Input: dimensioned drawing with shaded views. Units: mm. Origin: part minimum x, y, z. A direction names the side the tool comes from. Give positions to 0.01 mm unless a question says otherwise; leave off trailing zeros. Order: outer loops, then holes, each group sorted by start corner. A loop starts at its lowest first (then second) coordinate and runs counter-clockwise, first axis right, second up. Notation, with made-up numbers: (-25, 89.25) -> (9, 89.25) arc R24 cw to (9, 128.25) -> close; hole circle Ø6 at (4, -15). An arc over 180 degrees is marked (long way). One line per question, with ' | ' between items. Start each with the question number.
(1) Section C-C (z = 0.5). Return loops of the section in (x, y).
(2) Section B-B (y = 9.5). Return loops of the section in (x, z).
(3) Mould query, pull axis X, two halves, no side actions, for the marked faces 4, 5 and 6. Classes: +X half, -X half, draft (parallel to the pull), parting line (faces both ways), or undercut.
(4) Section A-A (z = 3). Return loops of the section in (x, y), then the cut area to 3 significant figures.
(5) Ray query, L1, parallel to X at y = 13.25, z = 2.25; L2, parallel to Z at x = 26.5, y = 9.75; L3, parallel to Y at x = 37, z = 1.35. Return the intervals inside material, ascending.
(6) First-contact query: pin 1 Ø2.5 at (x, z) = (2, 3.5) entering from -Y; pin 2 Ø1.5 at (x, y) = (28.5, 11.5) entering from +Z; pin 3 Ø6 at (x, y) = (32, 2) entering from +Z; pin 4 Ø2 at (x, z) = (43.5, 1.5) entering from -Y. Flat tips, straight axial feed; report the tip coordinate or a pass-through.
(7) Set-up query: the marked faces 1, 2 and 3. Return all of +Z, -Z, +X, -X, +Y, -Y with unobstructed straight access to the full face (end or side cutting, diameter ignored); none if empty.
(8) Section D-D (x = 15). Return loops of the section in (y, z), then the cut area to 3 significant figures.
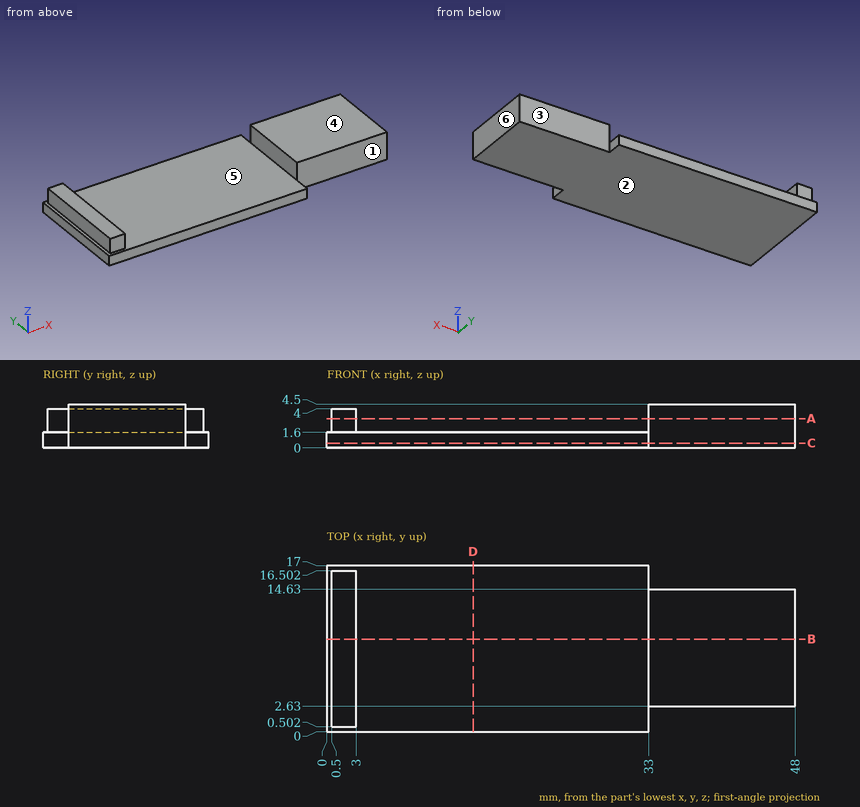
Response:
1) outline: (0, 0) -> (33, 0) -> (33, 2.63) -> (48, 2.63) -> (48, 14.63) -> (33, 14.63) -> (33, 17) -> (0, 17) -> close
2) outline: (0, 0) -> (48, 0) -> (48, 4.5) -> (33, 4.5) -> (33, 1.6) -> (3, 1.6) -> (3, 4) -> (0.5, 4) -> (0.5, 1.6) -> (0, 1.6) -> close
3) face 4: draft | face 5: undercut | face 6: +X half
4) outline: (0.5, 0.5) -> (3, 0.5) -> (3, 16.5) -> (0.5, 16.5) -> close; (33, 2.63) -> (48, 2.63) -> (48, 14.63) -> (33, 14.63) -> close | area: 220 mm^2
5) L1: x = 0.5 to 3, 33 to 48 | L2: z = 0 to 1.6 | L3: y = 2.63 to 14.63
6) pin 1: stops at y = 0.5 | pin 2: stops at z = 1.6 | pin 3: stops at z = 4.5 | pin 4: stops at y = 2.63
7) face 1: +Z, -Z, +X, -Y | face 2: -Z, +X, -X, +Y, -Y | face 3: +Z, -Z, +X, +Y
8) outline: (0, 0) -> (17, 0) -> (17, 1.6) -> (0, 1.6) -> close | area: 27.2 mm^2
